CAD build for the part. Positions are in the model's coordinates, mm. Face numbers are marked on the shaded views. Coordinates: 2 decimals unless noted, no trailing zeros. Loops run counter-clockwise (first coordinate to the right, second up) from the corner with the lowest first, then second, coordinate; pieces in that order, holes last. Notation, with made-up numbers: (53, 39) -> (112, 39) arc R31 ccw to (112, 75) -> close; hole circle Ø3 at (34, -35.75). An arc over 180 degrees is marked (long way). Write item = value, one per line. Start each with the question number.
(1) Band-saw the part on A-A (z = -40). Write the cut outline in (x, y), and give its area (3 significant figures).
(2) Drill centre lines: line 1 (X direction, y = 11, z = 5.25); line 2 (X direction, y = 5.5, z = -6.5). Where is each one in solid material? Low to high. Write a range as from..to.
(3) Band-saw the part on B-B (x = 35.5). Write the cut outline in (y, z), and give its area (3 significant figures).
(4) Pull direction Z, two halves, no side cores. Call the marked faces 1 and 2: +Z half, -Z half, draft (parallel to the pull), parting line (faces both ways), or undercut.
(5) Flat gauge pins, fed straight in: P1, Ø0.6, axis at x = -11.5, z = -7.5, coming from the -Y side; P2, Ø3, axis at x = -17, y = 12, coming from the +Z side; P3, Ø1.3, axis at x = 10.5, y = 11.5, coming from the +Z side; P4, Ø2, axis at y = 11.5, z = -4.5, coming from the -X side. Where does each tip first touch, or does it go through?
```python
from build123d import *

# Parameters (mm, degrees)
SKETCH1_W                = 200
SKETCH1_H                = 200
BOSS_EXTRUDE1_DEPTH      = 10
SHELL5_T                 = -3
BOSS_EXTRUDE2_DEPTH      = 13.75
SKETCH5_W                = 51.63175717
SKETCH5_H                = 2.8
CUT_EXTRUDE1_DEPTH       = 4.5
SKETCH6_W                = 5
SKETCH6_H                = 4.5
BOSS_EXTRUDE3_DEPTH      = 0.35
SKETCH7_W                = 3.5
SKETCH7_H                = 1
CUT_EXTRUDE2_DEPTH       = 3.5
F_2_0_2_DIAMETER_HOLE2_D = 2
FILLET1_R                = 10


with BuildPart() as part:
    # Sketch1 → Boss-Extrude1 (new body)
    with BuildSketch(Plane(origin=(0, 0, 0), x_dir=(1, 0, 0), z_dir=(0, 1, 0))):
        Rectangle(SKETCH1_W, SKETCH1_H)
    extrude(amount=BOSS_EXTRUDE1_DEPTH)

    # Shell5
    shell5_openings = [part.faces().sort_by_distance(p)[0] for p in [
        (0, 0, 0),
    ]]
    offset(amount=SHELL5_T, openings=shell5_openings, kind=Kind.INTERSECTION)

    # Sketch2 → Boss-Extrude2 (add, symmetric)
    with BuildSketch(Plane.XY):
        Polygon((-11.034760645, 10), (-11.034760645, 12.6), (-12.284760645, 12.6), (-12.284760645, 15.1), (-7.284760645, 15.1), (-7.284760645, 12.6), (-8.534760645, 12.6), (-8.534760645, 10), align=None)
        Polygon((8.965239355, 10), (11.465239355, 10), (11.465239355, 12.6), (12.715239355, 12.6), (12.715239355, 15.1), (7.715239355, 15.1), (7.715239355, 12.6), (8.965239355, 12.6), align=None)
    extrude(amount=BOSS_EXTRUDE2_DEPTH, both=True)

    # Sketch5 → Cut-Extrude1 (cut)
    with BuildSketch(Plane.XY.offset(13.75)):
        with Locations((-9.472877717, 13.7)):
            Rectangle(SKETCH5_W, SKETCH5_H)
        with Locations((17.311892559, -46.179704591)):
            Rectangle(SKETCH5_W, SKETCH5_H)
    extrude(amount=-CUT_EXTRUDE1_DEPTH, mode=Mode.SUBTRACT)

    # Sketch6 → Boss-Extrude3 (add)
    with BuildSketch(Plane(origin=(0, 12.3, 0), x_dir=(1, 0, 0), z_dir=(0, 1, 0))):
        with Locations((10.215239355, -11.5)):
            Rectangle(SKETCH6_W, SKETCH6_H)
        with Locations((-9.784760645, -11.5)):
            Rectangle(SKETCH6_W, SKETCH6_H)
    extrude(amount=BOSS_EXTRUDE3_DEPTH)

    # Sketch7 → Cut-Extrude2 (cut)
    with BuildSketch(Plane.XY.offset(9.25)):
        with Locations((10.215239355, 13.85)):
            Rectangle(SKETCH7_W, SKETCH7_H)
        with Locations((-9.784760645, 13.85)):
            Rectangle(SKETCH7_W, SKETCH7_H)
    extrude(amount=-CUT_EXTRUDE2_DEPTH, mode=Mode.SUBTRACT)

    # Ø2.0 (2) Diameter Hole2 (through all)
    with Locations(Plane(origin=(0, 15.1, 0), x_dir=(1, 0, 0), z_dir=(0, 1, 0))):
        with Locations((-9.784760645, -5.25), (10.215239355, -5.25)):
            Hole(F_2_0_2_DIAMETER_HOLE2_D / 2)

    # Fillet1
    fillet1_edges = [part.edges().sort_by_distance(p)[0] for p in [
        (-100, 5, -100),
        (100, 5, -100),
        (100, 5, 100),
        (-100, 5, 100),
    ]]
    fillet(fillet1_edges, radius=FILLET1_R)


solid = part.part
```
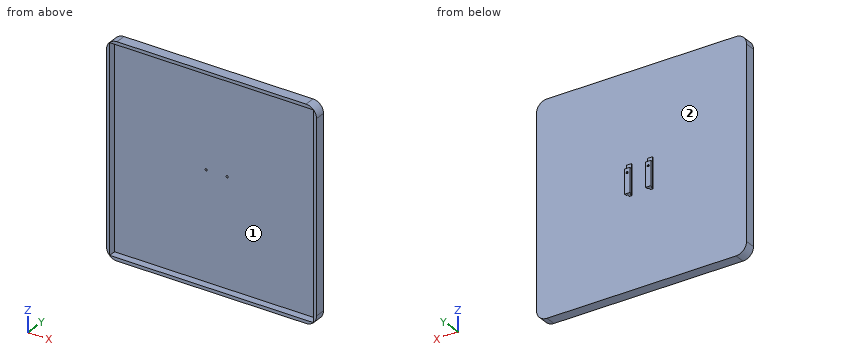
Findings below:
q1.outline = (-100, 0) -> (-97, 0) -> (-97, 7) -> (97, 7) -> (97, 0) -> (100, 0) -> (100, 10) -> (-100, 10) -> close
q1.area = 642 mm²
q2.line_1 = -11.03..-10.78, -8.78..-8.53, 8.97..9.22, 11.22..11.47
q2.line_2 = -100..-97, 97..100
q3.outline = (0, -100) -> (10, -100) -> (10, 100) -> (0, 100) -> (0, 97) -> (7, 97) -> (7, -97) -> (0, -97) -> close
q3.area = 642 mm²
q4.face_1 = undercut
q4.face_2 = draft
q5.P1 = 7
q5.P2 = through
q5.P3 = 13.75
q5.P4 = -11.03
